Here's how the part is built. I have some questions about the finished solid (model axes, mm). A direction names the side the tool comes from. Round coordinates to 2 decimals unless told otherwise and drop trailing zeros. Loops run counter-clockwise (first coordinate to the right, second up) from the corner with the lowest first, then second, coordinate; pieces in that order, holes last. Notation, with made-up numbers: M 29.5,77.5 L 52.5,77.5 A34 cw 52.5,115.5 Z; hole C 48.5,-1 d6. An arc over 180 degrees is marked long. Answer as a JSON object with one key per item and string values.
from build123d import *

# Parameters (mm, degrees)
SKETCH1_R           = 7
BOSS_EXTRUDE1_DEPTH = 0.5
SKETCH2_R           = 9.9
BOSS_EXTRUDE2_DEPTH = 1.3
SKETCH3_R           = 8.1
BOSS_EXTRUDE3_DEPTH = 11.2
SKETCH4_R           = 9.9
BOSS_EXTRUDE4_DEPTH = 1.3
SKETCH5_R           = 7
BOSS_EXTRUDE5_DEPTH = 0.5
SKETCH6_R           = 4
CUT_EXTRUDE1_DEPTH  = 21.373021376


with BuildPart() as part:
    # Sketch1 → Boss-Extrude1 (new body)
    with BuildSketch(Plane.XY):
        Circle(SKETCH1_R)
    extrude(amount=BOSS_EXTRUDE1_DEPTH)

    # Sketch2 → Boss-Extrude2 (add)
    with BuildSketch(Plane.XY.offset(0.5)):
        Circle(SKETCH2_R)
    extrude(amount=BOSS_EXTRUDE2_DEPTH)

    # Sketch3 → Boss-Extrude3 (add)
    with BuildSketch(Plane.XY.offset(1.8)):
        Circle(SKETCH3_R)
    extrude(amount=BOSS_EXTRUDE3_DEPTH)

    # Sketch4 → Boss-Extrude4 (add)
    with BuildSketch(Plane.XY.offset(13)):
        Circle(SKETCH4_R)
    extrude(amount=BOSS_EXTRUDE4_DEPTH)

    # Sketch5 → Boss-Extrude5 (add)
    with BuildSketch(Plane.XY.offset(14.3)):
        Circle(SKETCH5_R)
    extrude(amount=BOSS_EXTRUDE5_DEPTH)

    # Sketch6 → Cut-Extrude1 (cut, through all)
    with BuildSketch(Plane.XY.offset(14.8)):
        Circle(SKETCH6_R)
    extrude(amount=-CUT_EXTRUDE1_DEPTH, mode=Mode.SUBTRACT)


solid = part.part
Item 1: I want a section at D-D on x = -5.5. List the corners of the cut face in (y, z) for me.
Solution:
{"outline": "M -8.23,0.5 L -4.33,0.5 L -4.33,0 L 4.33,0 L 4.33,0.5 L 8.23,0.5 L 8.23,1.8 L 5.95,1.8 L 5.95,13 L 8.23,13 L 8.23,14.3 L 4.33,14.3 L 4.33,14.8 L -4.33,14.8 L -4.33,14.3 L -8.23,14.3 L -8.23,13 L -5.95,13 L -5.95,1.8 L -8.23,1.8 Z"}
Item 2: I want a section at C-C on z = 8. List the corners of the cut face in (x, y) for me, plus the area to 3 significant figures.
Solution:
{"outline": "C 0,0 d16.2; hole C 0,0 d8", "area": "156 mm2"}
Item 3: For faces 4 (the face through (2, 7, 0.5)), 5 (the face through (2, 7, 14.3)), 6 (the face through (-1.756, -7.907, 7.322)), which set-ups out of +Z, -Z, +X, -X, +Y, -Y let a thin tool reach every point of the face, with its end or its side?
Solution:
{"face 4": "-Z", "face 5": "+Z", "face 6": "none"}
Item 4: For P1, Ø6, axis at y = -4.5, z = 10.5, coming from the -X side; P2, Ø5, axis at x = 0, y = 0, coming from the -Z side; P3, Ø1, axis at x = -7.5, z = 9, coming from the +Y side; P4, Ø6, axis at y = -0.5, z = 8.5, coming from the +X side, each with a flat end and sliding along its axis, tell me the tip position at first contact or that it passes through.
Solution:
{"P1": "stops at x = -9.48", "P2": "passes through", "P3": "stops at y = 4.08", "P4": "stops at x = 8.1"}
Item 5: If I drill on L1, parallel to Y at x = 0, z = 3.75; L2, parallel to Z at x = 7, y = -6.5; L3, parallel to Y at x = -3, z = 13.25, over which ranges is the centre line in solid material (lowest first)? Write a range as from..to.
Solution:
{"L1": "y = -8.1..-4, 4..8.1", "L2": "z = 0.5..1.8, 13..14.3", "L3": "y = -9.43..-2.65, 2.65..9.43"}
Item 6: We'd pull the mould along X, two halves only. Please class faces 1 (the face through (-0.867, -3.905, 7.504)), 2 (the face through (-8.113, 1.513, 13)), 3 (the face through (9.443, 2.974, 1.141)): +X half, -X half, draft (parallel to the pull), parting line (faces both ways), or undercut.
Solution:
{"face 1": "undercut", "face 2": "draft", "face 3": "parting line"}
Item 7: I want a section at A-A on y = 0. List the corners of the cut face in (x, z) for me.
Solution:
{"outline": "M -9.9,0.5 L -7,0.5 L -7,0 L -4,0 L -4,14.8 L -7,14.8 L -7,14.3 L -9.9,14.3 L -9.9,13 L -8.1,13 L -8.1,1.8 L -9.9,1.8 Z; M 4,0 L 7,0 L 7,0.5 L 9.9,0.5 L 9.9,1.8 L 8.1,1.8 L 8.1,13 L 9.9,13 L 9.9,14.3 L 7,14.3 L 7,14.8 L 4,14.8 Z"}
